Verification items for this drawing (mm, ordinates from the low corner). Give positions to 0.01 mm unless a question says otherwise; leave off trailing zeros. Order: outer loops, then holes, each group sorted by start corner. A loop starts at its lowest first (then second) coordinate and runs counter-clockwise, first axis right, second up. Notation, with made-up numbers: M 58.25,44.25 L 83.25,44.25 A17 cw 83.25,64.25 Z; hole C 16,-31 d9. An arc over 180 degrees is marked long. Answer as a JSON object with one key per item and string values.
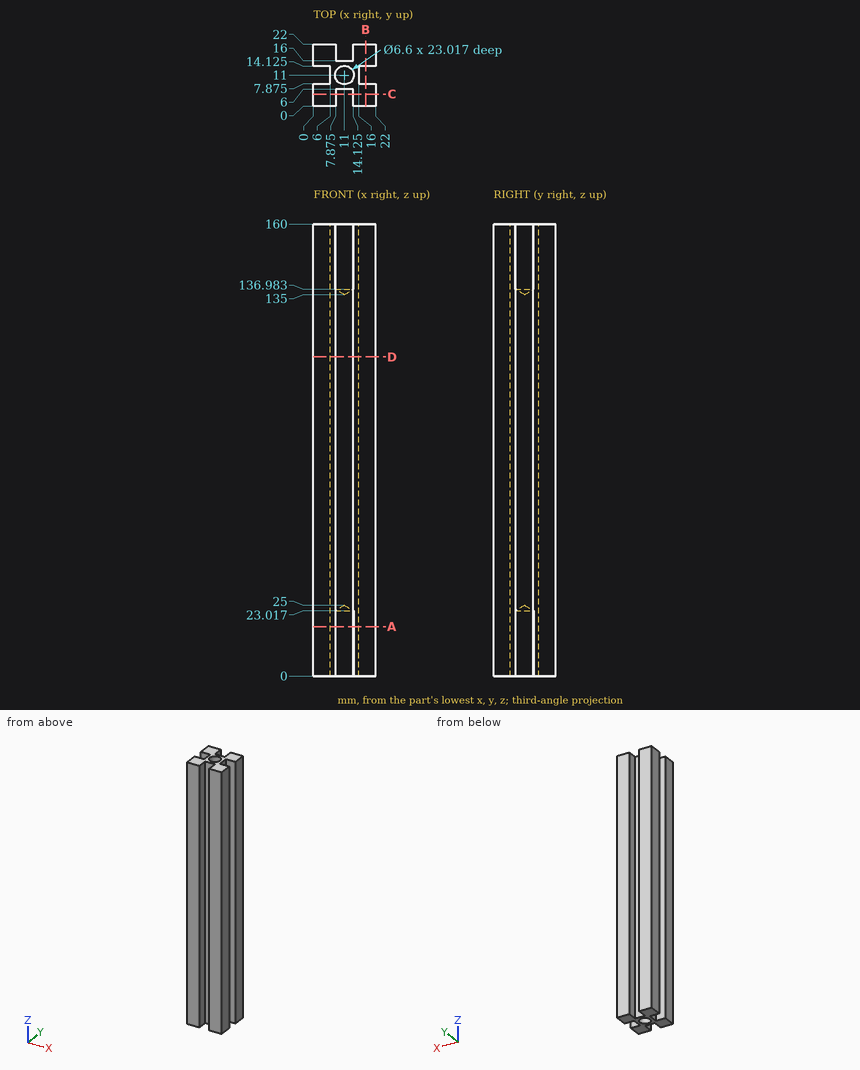
Q1. Material ranges on L1, parallel to X at y = 11, z = 14.25; L2, parallel to Y at x = 4, z = 152 (3 decimals), recorded low to high.
Resolved:
{"L1": "x = 6 to 7.7, 14.3 to 16", "L2": "y = 0 to 7.875, 14.125 to 22"}
Q2. Gauge pin test, flat ends, axial feed: pin 1 Ø3 at (y, z) = (10, 92) entering from -X; pin 2 Ø3 at (x, z) = (10, 89) entering from -Y; pin 3 Ø1.9 at (x, z) = (12, 64) entering from +Y. Record the tip position at first contact, or that the pin passes through.
Resolved:
{"pin 1": "stops at x = 6", "pin 2": "stops at y = 6", "pin 3": "stops at y = 16"}
Q3. Section check B-B on x = 18.5. Record the cut outline in (y, z) (3 decimals).
Resolved:
{"outline": "M 0,0 L 7.875,0 L 7.875,160 L 0,160 Z; M 14.125,0 L 22,0 L 22,160 L 14.125,160 Z"}
Q4. Section check A-A on z = 17.5. Record the cut outline in (x, y) (3 decimals).
Resolved:
{"outline": "M 0,0 L 7.875,0 L 7.875,6 L 14.125,6 L 14.125,0 L 22,0 L 22,7.875 L 16,7.875 L 16,14.125 L 22,14.125 L 22,22 L 14.125,22 L 14.125,16 L 7.875,16 L 7.875,22 L 0,22 L 0,14.125 L 6,14.125 L 6,7.875 L 0,7.875 Z; hole C 11,11 d6.6"}
Q5. Section check D-D on z = 113. Record the cut outline in (x, y) (3 decimals).
Resolved:
{"outline": "M 0,0 L 7.875,0 L 7.875,6 L 14.125,6 L 14.125,0 L 22,0 L 22,7.875 L 16,7.875 L 16,14.125 L 22,14.125 L 22,22 L 14.125,22 L 14.125,16 L 7.875,16 L 7.875,22 L 0,22 L 0,14.125 L 6,14.125 L 6,7.875 L 0,7.875 Z"}
